Could you check a few things on this model? Use its own coordinates, in mm. Give positions to 0.01 mm unless a question says otherwise; leave off trailing zeros. Loops run counter-clockwise (first coordinate to the right, second up) from the corner with the lowest first, then second, coordinate; pieces in that order, holes last. Notation, with made-up numbers: M 42.5,61 L 85.5,61 A18 ccw 85.5,76 Z; hole C -31,45.5 d8. An arc over 180 degrees is marked long. Answer in a Markdown table with one row per item. Add a question column.
1. If we section it at B-B on z = -17.5: List the corners of the cut face in (x, y) for me, then the cut area to 3 significant figures.
2. If we section it at A-A on x = 2.25: List the corners of the cut face in (y, z) for me.
3. I need wall thicknesses on line 1 along Y through (x, z) = (2.2, -23); line 2 along Z through (x, y) = (2.4, 37); line 3 along Y through (x, z) = (0.55, -4). Which ranges of each line are inside material? Lowest first, please. Write a range as from..to.
4. I'm going to push flat-ended pins straight in: pin 1 Ø0.9 at (x, z) = (1.5, -1) entering from -Y; pin 2 Ø1.5 at (x, z) = (1.5, -16) entering from -Y; pin 3 Ø0.9 at (x, z) = (1.5, -2) entering from +Y. Where does each tip first touch, or does it pass through?
5. If we section it at C-C on y = 23.5: List the corners of the cut face in (x, z) for me, then the cut area to 3 significant figures.
```python
from build123d import *

# Parameters (mm, degrees)
SKETCH_1_W          = 25
SKETCH_1_H          = 86
EXTRUDE_2_DEPTH     = 3
SKETCH_4_W          = 3
SKETCH_4_H          = 12
SKETCH_4_H_2        = 42
CUT_EXTRUDE_1_DEPTH = 4
SKETCH_5_W          = 7
SKETCH_5_H          = 3
CUT_EXTRUDE_2_DEPTH = 4


with BuildPart() as part:
    # 스케치1 → 보스-돌출2 (new body)
    with BuildSketch(Plane(origin=(0, 0, 0), x_dir=(0, 0, -1), z_dir=(1, 0, 0))):
        with Locations((12.5, 43)):
            Rectangle(SKETCH_1_W, SKETCH_1_H)
    extrude(amount=EXTRUDE_2_DEPTH)

    # 스케치4 → 컷-돌출1 (cut, through all)
    with BuildSketch(Plane(origin=(3, 0, 0), x_dir=(0, 0, -1), z_dir=(1, 0, 0))):
        with Locations((1.5, 80)):
            Rectangle(SKETCH_4_W, SKETCH_4_H)
        with Locations((23.5, 80)):
            Rectangle(SKETCH_4_W, SKETCH_4_H)
        with Locations((23.5, 6)):
            Rectangle(SKETCH_4_W, SKETCH_4_H)
        with Locations((1.5, 6)):
            Rectangle(SKETCH_4_W, SKETCH_4_H)
        with Locations((1.5, 43)):
            Rectangle(SKETCH_4_W, SKETCH_4_H_2)
        with Locations((23.5, 43)):
            Rectangle(SKETCH_4_W, SKETCH_4_H_2)
    extrude(amount=-CUT_EXTRUDE_1_DEPTH, mode=Mode.SUBTRACT)

    # 스케치5 → 컷-돌출2 (cut, through all)
    with BuildSketch(Plane(origin=(3, 0, 0), x_dir=(0, 0, -1), z_dir=(1, 0, 0))):
        with Locations((6.5, 84.5)):
            Rectangle(SKETCH_5_W, SKETCH_5_H)
        with Locations((18.5, 84.5)):
            Rectangle(SKETCH_5_W, SKETCH_5_H)
        with Locations((6.5, 1.5)):
            Rectangle(SKETCH_5_W, SKETCH_5_H)
        with Locations((18.5, 1.5)):
            Rectangle(SKETCH_5_W, SKETCH_5_H)
    extrude(amount=-CUT_EXTRUDE_2_DEPTH, mode=Mode.SUBTRACT)


solid = part.part
```
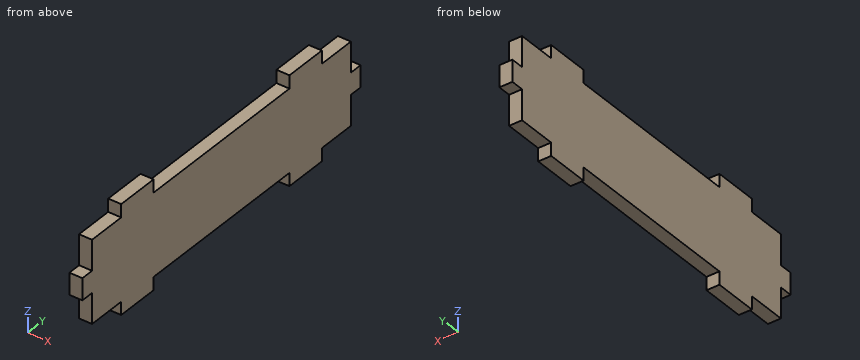
Results:
| question | item | result |
|---|---|---|
| 1 | outline | M 0,3 L 3,3 L 3,83 L 0,83 Z |
| 1 | area | 240 mm2 |
| 2 | outline | M 0,-15 L 3,-15 L 3,-22 L 12,-22 L 12,-25 L 22,-25 L 22,-22 L 64,-22 L 64,-25 L 74,-25 L 74,-22 L 83,-22 L 83,-15 L 86,-15 L 86,-10 L 83,-10 L 83,-3 L 74,-3 L 74,0 L 64,0 L 64,-3 L 22,-3 L 22,0 L 12,0 L 12,-3 L 3,-3 L 3,-10 L 0,-10 Z |
| 3 | line 1 | 12..22, 64..74 |
| 3 | line 2 | -22..-3 |
| 3 | line 3 | 3..83 |
| 4 | pin 1 | y = 12 |
| 4 | pin 2 | y = 3 |
| 4 | pin 3 | y = 74 |
| 5 | outline | M 0,-22 L 3,-22 L 3,-3 L 0,-3 Z |
| 5 | area | 57.0 mm2 |
